Design review of the part built by this model. Coordinates are the model's own, in mm. A direction names the side the tool comes from. Give positions to 0.01 mm unless a question says otherwise; leave off trailing zeros. Order: outer loops, then holes, each group sorted by start corner. A loop starts at its lowest first (then second) coordinate and runs counter-clockwise, first axis right, second up. Notation, with made-up numbers: (-27, 18) -> (19, 18) arc R13 ccw to (19, 41) -> close; hole circle Ø4 at (83.25, 75). An arc over 180 degrees is marked (long way). One line per item, written item: value. Start each with the question number.
1) Consider section C-C (x = 0). State the section outline as (y, z) points (3 decimals).
2) The part is to be moulded in two halves that separate along Z. For faces 1 (the face through (3, -3, 0)), 2 (the face through (-1.19, -0.06, -4.18)), 3 (the face through (2.6, -2.7, 3)), 4 (the face through (3, -3, 4)), say which applies: released by +Z, released by -Z, zero draft, split by the parting line, or undercut.
3) Consider section A-A (z = -1.25). State the section outline as (x, y) points (3 decimals), plus the area to 3 significant figures.
4) Wall thickness on line 1 along Y through (x, z) = (0, 0.25) (3 decimals); line 2 along X through (y, z) = (0, -2.75) (3 decimals): over which ranges is each line inside the solid? List them lowest first. Write a range as from..to.
5) For pin 1 (2 mm diameter, centred on x = 0.5, z = -5.5, fed in from +Y); pin 2 (1 mm diameter, centred on y = -2, z = -6, fed in from +X); pin 3 (4 mm diameter, centred on x = -1.5, z = -3.5, fed in from -Y), all flat-tipped, find the tip position at first contact; note any pin that passes through.
6) Tool access review of faces 5 (the face through (2.804, -2.853, -3.845)), 6 (the face through (2.7, 2.6, 3)), 7 (the face through (0, -1, -1)), 8 (the face through (-1, 1, -7.8)), 9 (the face through (2.853, 2.804, -3.845)): name each direction out of +Z, -Z, +X, -X, +Y, -Y from which nothing blocks a thin tool from reaching the whole face with its end or side.
7) Consider section D-D (x = -4.5). State the section outline as (y, z) points, plus the area to 3 significant figures.
8) Consider section B-B (y = 0). State the section outline as (x, z) points (3 decimals), plus the area to 3 significant figures.
from build123d import *

# Parameters (mm, degrees)
SKIZZE1_R                       = 6.7
SKIZZE1_R_2                     = 3.75
SKIZZE1_R_3                     = 4
AUFSATZ_LINEAR_AUSTRAGEN1_DEPTH = 4
SKIZZE1_4_R                     = 4
SKIZZE1_4_R_2                   = 3.75
SKIZZE1_4_R_3                   = 1
AUFSATZ_LINEAR_AUSTRAGEN2_DEPTH = 7.8
SKIZZE1_6_R                     = 4
SKIZZE1_6_R_2                   = 1
AUFSATZ_LINEAR_AUSTRAGEN3_DEPTH = 2
M2_GEWINDEBOHRUNG1_D            = 1.6
M3_GEWINDEBOHRUNG1_D            = 2.5


with BuildPart() as part:
    # Skizze1 → Aufsatz-Linear austragen1 (new body)
    with BuildSketch(Plane.XY):
        Circle(SKIZZE1_R)
        Circle(SKIZZE1_R_2, mode=Mode.SUBTRACT)
        Circle(SKIZZE1_R_3)
        Circle(SKIZZE1_R_2, mode=Mode.SUBTRACT)
    extrude(amount=AUFSATZ_LINEAR_AUSTRAGEN1_DEPTH)

    # Skizze1_4 → Aufsatz-Linear austragen2 (add)
    with BuildSketch(Plane.XY):
        Circle(SKIZZE1_4_R)
        Circle(SKIZZE1_4_R_2, mode=Mode.SUBTRACT)
        Circle(SKIZZE1_4_R_2)
        Circle(SKIZZE1_4_R_3, mode=Mode.SUBTRACT)
    extrude(amount=-AUFSATZ_LINEAR_AUSTRAGEN2_DEPTH)

    # Skizze1_6 → Aufsatz-Linear austragen3 (add)
    with BuildSketch(Plane.XY):
        Circle(SKIZZE1_6_R)
        Circle(SKIZZE1_6_R_2, mode=Mode.SUBTRACT)
    extrude(amount=AUFSATZ_LINEAR_AUSTRAGEN3_DEPTH)

    # M2 Gewindebohrung1 (through all)
    with Locations(Plane.XY.offset(4)):
        with Locations((4.425, 0), (0, -4.425), (-4.425, 0), (0, 4.425)):
            Hole(M2_GEWINDEBOHRUNG1_D / 2)

    # M3 Gewindebohrung1 (through all)
    with Locations(Plane(origin=(0, 3.625, -3.8), x_dir=(1, 0, 0), z_dir=(0, 1, 0))):
        with Locations((0, 0)):
            Hole(M3_GEWINDEBOHRUNG1_D / 2)


solid = part.part
Checked values:
1. outline: (-6.7, 0) -> (-5.225, 0) -> (-5.225, 4) -> (-6.7, 4) -> close; (-3.625, -7.8) -> (-1, -7.8) -> (-1, -5.05) -> (-3.625, -5.05) -> close; (-3.625, -2.55) -> (-1, -2.55) -> (-1, 2) -> (-3.625, 2) -> close; (1, -7.8) -> (3.625, -7.8) -> (3.625, -5.05) -> (1, -5.05) -> close; (1, -2.55) -> (3.625, -2.55) -> (3.625, 2) -> (1, 2) -> close; (5.225, 0) -> (6.7, 0) -> (6.7, 4) -> (5.225, 4) -> close
2. face 1: released by -Z
2. face 2: undercut
2. face 3: zero draft
2. face 4: released by +Z
3. outline: (-3.948, -0.642) arc R4 ccw to (-0.642, -3.948) arc R0.8 cw to (0.642, -3.948) arc R4 ccw to (3.948, -0.642) arc R0.8 cw to (3.948, 0.642) arc R4 ccw to (0.642, 3.948) arc R0.8 cw to (-0.642, 3.948) arc R4 ccw to (-3.948, 0.642) arc R0.8 cw to start; hole circle Ø2 at (0, 0)
3. area: 45.8 mm^2
4. line 1: y = -6.7..-5.225, -3.625..-1, 1..3.625, 5.225..6.7
4. line 2: x = -3.625..-1, 1..3.625
5. pin 1: stops at y = 3.95
5. pin 2: stops at x = 3.71
5. pin 3: stops at y = -3.95
6. face 5: -Z, +X, -Y
6. face 6: +Z
6. face 7: +Z, -Z
6. face 8: -Z, +X, -X, +Y, -Y
6. face 9: -Z, +X, +Y
7. outline: (-4.96, 0) -> (-0.8, 0) -> (-0.8, 4) -> (-4.96, 4) -> close; (0.8, 0) -> (4.96, 0) -> (4.96, 4) -> (0.8, 4) -> close
7. area: 33.3 mm^2
8. outline: (-6.7, 0) -> (-5.225, 0) -> (-5.225, 4) -> (-6.7, 4) -> close; (-3.625, -7.8) -> (-1, -7.8) -> (-1, -4.55) arc R1.25 cw to (-1, -3.05) -> (-1, 2) -> (-3.625, 2) -> close; (1, -7.8) -> (3.625, -7.8) -> (3.625, 2) -> (1, 2) -> (1, -3.05) arc R1.25 cw to (1, -4.55) -> close; (5.225, 0) -> (6.7, 0) -> (6.7, 4) -> (5.225, 4) -> close
8. area: 62.7 mm^2
